Verification items for the finished model (mm, model axes). Give positions to 0.01 mm unless a question says otherwise; leave off trailing zeros. Loops run counter-clockwise (first coordinate to the right, second up) from the corner with the lowest first, then second, coordinate; pieces in that order, holes last. Notation, with made-up numbers: M 19,89.25 L 31,89.25 A22 cw 31,101.25 Z; hole C 12,85.5 d6. An arc over 180 degrees is marked long. Use CSV: the item, a comma, the result in double quotes.
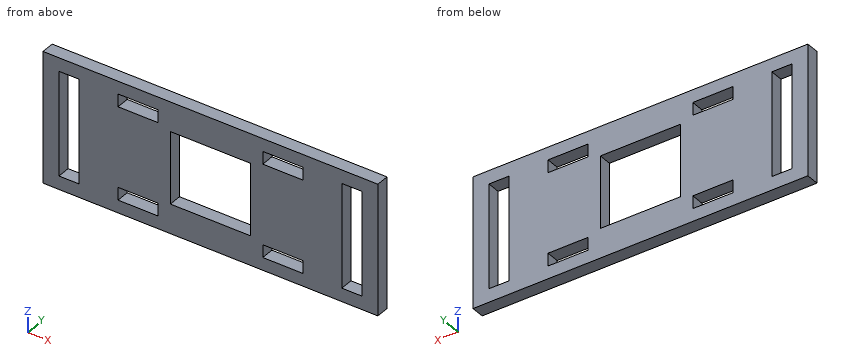
from build123d import *

# Parameters (mm, degrees)
SKETCH1_W           = 83.65
SKETCH1_H           = 32.7
SKETCH1_W_2         = 5
SKETCH1_H_2         = 26
SKETCH1_W_3         = 10
SKETCH1_H_3         = 3.175
SKETCH1_W_4         = 20
SKETCH1_H_4         = 18
BOSS_EXTRUDE1_DEPTH = 3.25


with BuildPart() as part:
    # Sketch1 → Boss-Extrude1 (new body)
    with BuildSketch(Plane(origin=(0, 0, 0), x_dir=(1, 0, 0), z_dir=(0, 1, 0))):
        Rectangle(SKETCH1_W, SKETCH1_H)
        with Locations((-35.325, 0)):
            Rectangle(SKETCH1_W_2, SKETCH1_H_2, mode=Mode.SUBTRACT)
        with Locations((-18.075, 11.5875)):
            Rectangle(SKETCH1_W_3, SKETCH1_H_3, mode=Mode.SUBTRACT)
        with Locations((35.325, 0)):
            Rectangle(SKETCH1_W_2, SKETCH1_H_2, mode=Mode.SUBTRACT)
        with Locations((18.075, 11.5875)):
            Rectangle(SKETCH1_W_3, SKETCH1_H_3, mode=Mode.SUBTRACT)
        with Locations((18.075, -11.5875)):
            Rectangle(SKETCH1_W_3, SKETCH1_H_3, mode=Mode.SUBTRACT)
        with Locations((-18.075, -11.5875)):
            Rectangle(SKETCH1_W_3, SKETCH1_H_3, mode=Mode.SUBTRACT)
        Rectangle(SKETCH1_W_4, SKETCH1_H_4, mode=Mode.SUBTRACT)
    extrude(amount=BOSS_EXTRUDE1_DEPTH)


solid = part.part
(1) Section check B-B on z = 11.5. Record the cut outline in (x, y) (3 decimals).
Calculated:
outline,"M -41.825,0 L -37.825,0 L -37.825,3.25 L -41.825,3.25 Z; M -32.825,0 L -23.075,0 L -23.075,3.25 L -32.825,3.25 Z; M -13.075,0 L 13.075,0 L 13.075,3.25 L -13.075,3.25 Z; M 23.075,0 L 32.825,0 L 32.825,3.25 L 23.075,3.25 Z; M 37.825,0 L 41.825,0 L 41.825,3.25 L 37.825,3.25 Z"
(2) Section check A-A on x = -36. Record the cut outline in (y, z).
Calculated:
outline,"M 0,-16.35 L 3.25,-16.35 L 3.25,-13 L 0,-13 Z; M 0,13 L 3.25,13 L 3.25,16.35 L 0,16.35 Z"
(3) Section check C-C on y = 2. Count the separate pieces of the cut face and the enclosed holes in it, plus the area to 3 significant figures.
Calculated:
separate pieces,"1"
enclosed holes,"7"
area,"1,990 mm²"
(4) Scan lines: L1, parallel to Z at x = 16, y = 1.05 (3 decimals); L2, parallel to X at y = 2.7, z = -2 (3 decimals); L3, parallel to X at y = 2.95, z = -9.5 (3 decimals). Record each from-to range of solid material in increasing order. Write a range as from..to.
Calculated:
L1,"z = -16.35..-13.175, -10..10, 13.175..16.35"
L2,"x = -41.825..-37.825, -32.825..-10, 10..32.825, 37.825..41.825"
L3,"x = -41.825..-37.825, -32.825..32.825, 37.825..41.825"
(5) Section check D-D on z = 7.5. Record the cut outline in (x, y) (3 decimals), plus the area to 3 significant figures.
Calculated:
outline,"M -41.825,0 L -37.825,0 L -37.825,3.25 L -41.825,3.25 Z; M -32.825,0 L -10,0 L -10,3.25 L -32.825,3.25 Z; M 10,0 L 32.825,0 L 32.825,3.25 L 10,3.25 Z; M 37.825,0 L 41.825,0 L 41.825,3.25 L 37.825,3.25 Z"
area,"174 mm²"
